Check sheet for the modelled part. Datum: model origin and axes. Units: mm. Round coordinates to 2 decimals unless told otherwise and drop trailing zeros. Write each loop counter-clockwise with the first axis right and the second up, starting at its lowest first coordinate (ties: lowest second). Pieces come first, ordered by that corner, then holes.
Item 1: Section check B-B, the plane x = 38. Record the cut outline in (y, z), plus the area to 3 significant figures.
Item 2: Depth check by flat-ended pin: pin 1 (2 mm diameter, centred on x = 63, z = 4, fed in from +Y); pin 2 (1 mm diameter, centred on x = -1, z = 1, fed in from -Y); pin 3 (0.6 mm diameter, centred on y = 81.5, z = 1, fed in from -X); pin 4 (1.3 mm diameter, centred on x = 84, z = 1, fed in from +Y). Enter the tip coordinate at first touch or a pass-through.
Item 3: Section check A-A, the plane y = 35. Record the cut outline in (x, z), plus the area to 3 significant figures.
Item 4: Section check C-C, the plane y = 69.5. Record the cut outline in (x, z).
Item 5: Section check D-D, the plane z = 3.25. Record the cut outline in (x, y).
Item 6: Material ranges on line 1 along X through (y, z) = (70.5, 0.75); line 2 along Y through (x, z) = (7, 0.75); line 3 along X through (y, z) = (-6, 6.25), recorded low to high.
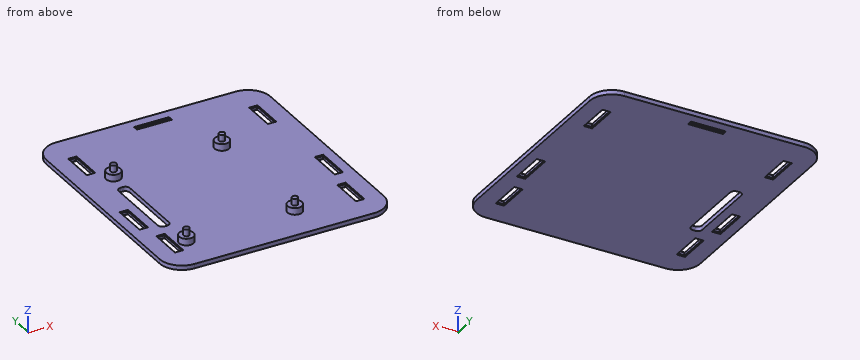
from build123d import *

# Parameters (mm, degrees)
SKETCH1_W           = 101
SKETCH1_H           = 110
BOSS_EXTRUDE1_DEPTH = 2
SKETCH3_W           = 15
SKETCH3_H           = 1.5
SKETCH3_W_2         = 3
SKETCH3_H_2         = 15
CUT_EXTRUDE1_DEPTH  = 128.433943673
SKETCH7_R           = 3.25
BOSS_EXTRUDE2_DEPTH = 3
SKETCH8_R           = 1.3
BOSS_EXTRUDE3_DEPTH = 3
CHAMFER2_SIZE       = 0.4
SKETCH9_W           = 3
SKETCH9_H           = 14
CUT_EXTRUDE2_DEPTH  = 5
CHAMFER3_SIZE       = 0.4
SKETCH10_W          = 5
SKETCH10_H          = 35
CUT_EXTRUDE3_DEPTH  = 128.559437126
FILLET1_R           = 2
FILLET2_R           = 10


with BuildPart() as part:
    # Sketch1 → Boss-Extrude1 (new body)
    with BuildSketch(Plane.XY):
        with Locations((42.5, 32.1)):
            Rectangle(SKETCH1_W, SKETCH1_H)
    extrude(amount=BOSS_EXTRUDE1_DEPTH)

    # Sketch3 → Cut-Extrude1 (cut, through all)
    with BuildSketch(Plane.XY.offset(2)):
        with Locations((42.5, 81.35)):
            Rectangle(SKETCH3_W, SKETCH3_H)
        with Locations((-1.5, 19.1)):
            Rectangle(SKETCH3_W_2, SKETCH3_H_2)
        with Locations((86.5, 19.1)):
            Rectangle(SKETCH3_W_2, SKETCH3_H_2)
    extrude(amount=-CUT_EXTRUDE1_DEPTH, mode=Mode.SUBTRACT)

    # Sketch7 → Boss-Extrude2 (add)
    with BuildSketch(Plane.XY.offset(2)):
        with Locations(Location((8.05, 52.05, 0), (0, 0, 180))):
            Circle(SKETCH7_R)
        with Locations(Location((56.95, 52.05, 0), (0, 0, 180))):
            Circle(SKETCH7_R)
        with Locations(Location((8.05, -5.85, 0), (0, 0, 180))):
            Circle(SKETCH7_R)
        with Locations(Location((56.95, -5.85, 0), (0, 0, 180))):
            Circle(SKETCH7_R)
    extrude(amount=BOSS_EXTRUDE2_DEPTH)

    # Sketch8 → Boss-Extrude3 (add)
    with BuildSketch(Plane.XY.offset(5)):
        with Locations(Location((8.05, -5.85, 0), (0, 0, 180))):
            Circle(SKETCH8_R)
        with Locations(Location((56.95, -5.85, 0), (0, 0, 180))):
            Circle(SKETCH8_R)
        with Locations(Location((56.95, 52.05, 0), (0, 0, 180))):
            Circle(SKETCH8_R)
        with Locations(Location((8.05, 52.05, 0), (0, 0, 180))):
            Circle(SKETCH8_R)
    extrude(amount=BOSS_EXTRUDE3_DEPTH)

    # Chamfer2
    chamfer2_edges = [part.edges().sort_by_distance(p)[0] for p in [
        (35, 81.35, 0),
        (42.5, 82.1, 0),
        (50, 81.35, 0),
        (42.5, 80.6, 0),
        (35, 81.35, 2),
        (42.5, 80.6, 2),
        (50, 81.35, 2),
        (42.5, 82.1, 2),
        (-3, 19.1, 0),
        (-1.5, 26.6, 0),
        (0, 19.1, 0),
        (-1.5, 11.6, 0),
        (-3, 19.1, 2),
        (-1.5, 11.6, 2),
        (0, 19.1, 2),
        (-1.5, 26.6, 2),
        (85, 19.1, 0),
        (86.5, 26.6, 0),
        (88, 19.1, 0),
        (86.5, 11.6, 0),
        (85, 19.1, 2),
        (86.5, 11.6, 2),
        (88, 19.1, 2),
        (86.5, 26.6, 2),
    ]]
    chamfer(chamfer2_edges, length=CHAMFER2_SIZE)

    # Sketch9 → Cut-Extrude2 (cut)
    with BuildSketch(Plane(origin=(0, 0, 0), x_dir=(-1, 0, 0), z_dir=(0, 0, -1))):
        with Locations((-83.3, -3.9)):
            Rectangle(SKETCH9_W, SKETCH9_H)
        with Locations((-83.3, 66.1)):
            Rectangle(SKETCH9_W, SKETCH9_H)
        with Locations((-1.7, -3.9)):
            Rectangle(SKETCH9_W, SKETCH9_H)
        with Locations((-1.7, 66.1)):
            Rectangle(SKETCH9_W, SKETCH9_H)
    extrude(amount=-CUT_EXTRUDE2_DEPTH, mode=Mode.SUBTRACT)

    # Chamfer3
    chamfer3_edges = [part.edges().sort_by_distance(p)[0] for p in [
        (84.8, -3.9, 2),
        (83.3, 3.1, 2),
        (81.8, -3.9, 2),
        (83.3, -10.9, 2),
        (84.8, -3.9, 0),
        (83.3, -10.9, 0),
        (81.8, -3.9, 0),
        (83.3, 3.1, 0),
        (84.8, 66.1, 2),
        (83.3, 73.1, 2),
        (81.8, 66.1, 2),
        (83.3, 59.1, 2),
        (84.8, 66.1, 0),
        (83.3, 59.1, 0),
        (81.8, 66.1, 0),
        (83.3, 73.1, 0),
        (3.2, -3.9, 2),
        (1.7, 3.1, 2),
        (0.2, -3.9, 2),
        (1.7, -10.9, 2),
        (3.2, -3.9, 0),
        (1.7, -10.9, 0),
        (0.2, -3.9, 0),
        (1.7, 3.1, 0),
        (3.2, 66.1, 2),
        (1.7, 73.1, 2),
        (0.2, 66.1, 2),
        (1.7, 59.1, 2),
        (3.2, 66.1, 0),
        (1.7, 59.1, 0),
        (0.2, 66.1, 0),
        (1.7, 73.1, 0),
    ]]
    chamfer(chamfer3_edges, length=CHAMFER3_SIZE)

    # Sketch10 → Cut-Extrude3 (cut, through all)
    with BuildSketch(Plane.XY.offset(2)):
        with Locations((7, 26.1)):
            Rectangle(SKETCH10_W, SKETCH10_H)
    extrude(amount=-CUT_EXTRUDE3_DEPTH, mode=Mode.SUBTRACT)

    # Fillet1
    fillet1_edges = [part.edges().sort_by_distance(p)[0] for p in [
        (4.5, 8.6, 1),
        (4.5, 43.6, 1),
        (9.5, 43.6, 1),
        (9.5, 8.6, 1),
    ]]
    fillet(fillet1_edges, radius=FILLET1_R)

    # Fillet2
    fillet2_edges = [part.edges().sort_by_distance(p)[0] for p in [
        (-8, 87.1, 1),
        (93, 87.1, 1),
        (93, -22.9, 1),
        (-8, -22.9, 1),
    ]]
    fillet(fillet2_edges, radius=FILLET2_R)


solid = part.part
Values found:
1. outline: (-22.9, 0) - (80.2, 0) - (80.6, 0.4) - (80.6, 1.6) - (80.2, 2) - (-22.9, 2) - close; (82.1, 0.4) - (82.5, 0) - (87.1, 0) - (87.1, 2) - (82.5, 2) - (82.1, 1.6) - close
1. area: 217 mm2
2. pin 1: passes through
2. pin 2: stops at y = -22.58
2. pin 3: stops at x = -7.12
2. pin 4: stops at y = 87.09
3. outline: (-8, 0) - (4.5, 0) - (4.5, 2) - (-8, 2) - close; (9.5, 0) - (93, 0) - (93, 2) - (9.5, 2) - close
3. area: 192 mm2
4. outline: (-8, 0) - (-0.2, 0) - (0.2, 0.4) - (0.2, 1.6) - (-0.2, 2) - (-8, 2) - close; (3.2, 0.4) - (3.6, 0) - (81.4, 0) - (81.8, 0.4) - (81.8, 1.6) - (81.4, 2) - (3.6, 2) - (3.2, 1.6) - close; (84.8, 0.4) - (85.2, 0) - (93, 0) - (93, 2) - (85.2, 2) - (84.8, 1.6) - close
5. outline: circle Ø6.5 at (8.05, -5.85); circle Ø6.5 at (8.05, 52.05); circle Ø6.5 at (56.95, -5.85); circle Ø6.5 at (56.95, 52.05)
6. line 1: x = -8 to 0.2, 3.2 to 81.8, 84.8 to 93
6. line 2: y = -22.9 to 8.6, 43.6 to 87.1
6. line 3: x = 6.76 to 9.34, 55.66 to 58.24
